from build123d import *

# Parameters (mm, degrees)
DODANIE_WYCI_GNI_CIE1_DEPTH = 1.5
SZKIC1_4_R                  = 2.5
DODANIE_WYCI_GNI_CIE2_DEPTH = 22.5
SZKIC3_R                    = 1.55
WYTNIJ_WYCI_GNI_CIE2_DEPTH  = 1.2
SZKIC1_5_R                  = 2
DODANIE_WYCI_GNI_CIE3_DEPTH = 11
SZKIC2_R                    = 0.85
WYTNIJ_WYCI_GNI_CIE3_DEPTH  = 9


with BuildPart() as part:
    # Szkic1 → Dodanie-wyci_gni_cie1 (new body)
    with BuildSketch(Plane(origin=(0, 0, 0), x_dir=(1, 0, 0), z_dir=(0, 1, 0))):
        with BuildLine():
            Line((16.795, -19.295), (-16.795, -19.295))
            ThreePointArc((-16.795, -19.295), (-18.562766953, -18.562766953), (-19.295, -16.795))
            Line((-19.295, -16.795), (-19.295, 16.795))
            ThreePointArc((-19.295, 16.795), (-18.562766953, 18.562766953), (-16.795, 19.295))
            Line((-16.795, 19.295), (16.795, 19.295))
            ThreePointArc((16.795, 19.295), (18.562766953, 18.562766953), (19.295, 16.795))
            Line((19.295, 16.795), (19.295, -16.795))
            ThreePointArc((19.295, -16.795), (18.562766953, -18.562766953), (16.795, -19.295))
        make_face()
    extrude(amount=DODANIE_WYCI_GNI_CIE1_DEPTH)

    # Szkic1_4 → Dodanie-wyci_gni_cie2 (add)
    with BuildSketch(Plane(origin=(0, 0, 0), x_dir=(1, 0, 0), z_dir=(0, 1, 0))):
        with Locations(Location((13.295, 7, 0), (0, 0, 90))):
            Circle(SZKIC1_4_R)
        with Locations(Location((-13.295, 7, 0), (0, 0, 90))):
            Circle(SZKIC1_4_R)
        with Locations(Location((13.295, -7, 0), (0, 0, 90))):
            Circle(SZKIC1_4_R)
        with Locations(Location((-13.295, -7, 0), (0, 0, 90))):
            Circle(SZKIC1_4_R)
    extrude(amount=DODANIE_WYCI_GNI_CIE2_DEPTH)

    # Szkic3 → Wytnij-wyci_gni_cie2 (cut)
    with BuildSketch(Plane.XZ.offset(-1.5)):
        with Locations(Location((0, 0, 0), (0, 0, 270))):
            Circle(SZKIC3_R)
    extrude(amount=WYTNIJ_WYCI_GNI_CIE2_DEPTH, mode=Mode.SUBTRACT)

    # Szkic1_5 → Dodanie-wyci_gni_cie3 (add)
    with BuildSketch(Plane(origin=(0, 0, 0), x_dir=(1, 0, 0), z_dir=(0, 1, 0))):
        with Locations(Location((13.965358928, -13.965358928, 0), (0, 0, 270))):
            Circle(SZKIC1_5_R)
        with Locations(Location((-13.965358928, 13.965358928, 0), (0, 0, 270))):
            Circle(SZKIC1_5_R)
    extrude(amount=-DODANIE_WYCI_GNI_CIE3_DEPTH)

    # Szkic2 → Wytnij-wyci_gni_cie3 (cut)
    with BuildSketch(Plane(origin=(0, -11, 0), x_dir=(1, 0, 0), z_dir=(0, 1, 0))):
        with Locations(Location((-14, 14, 0), (0, 0, 270))):
            Circle(SZKIC2_R)
        with Locations(Location((14, -14, 0), (0, 0, 270))):
            Circle(SZKIC2_R)
    extrude(amount=WYTNIJ_WYCI_GNI_CIE3_DEPTH, mode=Mode.SUBTRACT)


solid = part.part
Input: part model. Units: mm. Frame: model coordinates. A direction names the side the tool comes from. Round coordinates to 2 decimals unless told otherwise and drop trailing zeros. Write each loop counter-clockwise with the first axis right and the second up, starting at its lowest first coordinate (ties: lowest second). Pieces come first, ordered by that corner, then holes.
1) Reachability of faces 1 (the flat face through (-4, 1.5, 0)), 2 (the flat face through (-14, -2, -14)), 3 (the flat face through (-13, 22.5, -7)) from +Z, -Z, +X, -X, +Y, -Y: full face, straight path, thin tool, end or side. Return the list, or none.
2) Contact query for flat-ended pins moving along their axis: P1, Ø1, axis at y = 16, z = 6, coming from the -X side; P2, Ø3.5, axis at x = 0, z = 0, coming from the +Y side; P3, Ø2, axis at x = 14, z = 14, coming from the -Y side; P4, Ø3, axis at y = -2.5, z = 11.5, coming from the +X side. Output: stop coordinate, or through.
3) Cut plane D-D (y = 13). Return the cut outline in (x, z) (3 decimals).
4) Ray query, L1, parallel to X at y = -8.25, z = -14; L2, parallel to Y at x = 14, z = 15.5; L3, parallel to Y at x = 8, z = 12. Return the intervals inside material, ascending.
5) Cut plane A-A (x = 0). Return the cut outline in (y, z) (3 decimals), then the cut area to 3 significant figures.
6) Cut plane B-B (z = 0). Return the cut outline in (x, y) (3 decimals).
7) Draft query along Z for faces 4 (the cylindrical face through (14.26, -6.56, 14.81)), 5 (the flat face through (0, 1, 19.295)), 6 (the flat face through (-13, 22.5, 7)). Return one class per face: pulls with the +Z half, pulls with the -Z half, needs draft (parallel to the pull), parting line crosses it, or undercut.
8) Cut plane C-C (z = 7). Return the cut outline in (x, y) (3 decimals), then the cut area to 3 significant figures.
Geometry says:
1. face 1: +Y
1. face 2: -Y
1. face 3: +Z, -Z, +X, -X, +Y
2. P1: stops at x = -15.74
2. P2: stops at y = 1.5
2. P3: stops at y = -11
2. P4: stops at x = 15.72
3. outline: circle Ø5 at (-13.295, -7); circle Ø5 at (-13.295, 7); circle Ø5 at (13.295, -7); circle Ø5 at (13.295, 7)
4. L1: x = -15.97 to -14.85, -13.15 to -11.97
4. L2: y = -11 to 1.5
4. L3: y = 0 to 1.5
5. outline: (0, -19.295) - (1.5, -19.295) - (1.5, -1.55) - (0.3, -1.55) - (0.3, 1.55) - (1.5, 1.55) - (1.5, 19.295) - (0, 19.295) - close
5. area: 54.2 mm2
6. outline: (-19.295, 0) - (19.295, 0) - (19.295, 1.5) - (1.55, 1.5) - (1.55, 0.3) - (-1.55, 0.3) - (-1.55, 1.5) - (-19.295, 1.5) - close
7. face 4: undercut
7. face 5: pulls with the +Z half
7. face 6: needs draft
8. outline: (-19.295, 0) - (19.295, 0) - (19.295, 1.5) - (15.795, 1.5) - (15.795, 22.5) - (10.795, 22.5) - (10.795, 1.5) - (-10.795, 1.5) - (-10.795, 22.5) - (-15.795, 22.5) - (-15.795, 1.5) - (-19.295, 1.5) - close
8. area: 268 mm2
